```python
from build123d import *

# Parameters (mm, degrees)
F1_W     = 450
F1_H     = 450
F2_DEPTH = 25
F3_W     = 50
F3_H     = 50
F4_DEPTH = 450
F6_DEPTH = 25
F8_DEPTH = 25


with BuildPart() as f2:
    # F1 (on offset) → F2 (new body)
    with BuildSketch(Plane.XY.offset(450)):
        Rectangle(F1_W, F1_H)
    extrude(amount=F2_DEPTH)

    # F3 (on face) → F4 (join, through all)
    with BuildSketch(Plane(origin=(0, 0, 450), x_dir=(1, 0, 0), z_dir=(0, 0, -1))):
        with Locations((-200, -200)):
            Rectangle(F3_W, F3_H)
        with Locations((-200, 200)):
            Rectangle(F3_W, F3_H)
        with Locations((200, -200)):
            Rectangle(F3_W, F3_H)
        with Locations((200, 200)):
            Rectangle(F3_W, F3_H)
    extrude(amount=F4_DEPTH)

    # F5 (on face) → F6 (join)
    with BuildSketch(Plane.XZ.offset(225)):
        with BuildLine():
            Line((-277.210476888, 871.5779445495), (-225, 475))
            Line((-225, 475), (-174.568551971, 475))
            Line((-174.568551971, 475), (-219.5097934393, 816.3626197141))
            ThreePointArc((-219.5097934393, 816.3626197141), (0, 864.4554478408), (219.5097934393, 816.3626197141))
            Line((219.5097934393, 816.3626197141), (174.568551971, 475))
            Line((174.568551971, 475), (225, 475))
            Line((225, 475), (277.210476888, 871.5779445495))
            ThreePointArc((277.210476888, 871.5779445495), (0, 939.4554478408), (-277.210476888, 871.5779445495))
        make_face()
    extrude(amount=-F6_DEPTH)

    # F7 (on face) → F8 (join)
    with BuildSketch(Plane.XZ.offset(225)):
        with BuildLine():
            ThreePointArc((12.5, 864.3066172212), (0, 864.4554478408), (-12.5, 864.3066172212))
            Line((-12.5, 864.3066172212), (-12.5, 475))
            Line((-12.5, 475), (12.5, 475))
            Line((12.5, 475), (12.5, 864.3066172212))
        make_face()
        with BuildLine():
            Line((-140.2890822889, 871.5293721566), (-112.561047452, 475))
            Line((-112.561047452, 475), (-87.5, 475))
            Line((-87.5, 475), (-115.6574592783, 877.6704277765))
            ThreePointArc((-115.6574592783, 877.6704277765), (-127.9664582867, 874.5725752089), (-140.2890822889, 871.5293721566))
        make_face()
        with BuildLine():
            Line((87.5, 475), (112.561047452, 475))
            Line((112.561047452, 475), (140.2890822889, 871.5293721566))
            ThreePointArc((140.2890822889, 871.5293721566), (127.9664582867, 874.5725752089), (115.6574592783, 877.6704277765))
            Line((115.6574592783, 877.6704277765), (87.5, 475))
        make_face()
    extrude(amount=-F8_DEPTH)


solid = f2.part
```
Part model, mm, in its own coordinate system. A direction names the side the tool comes from. Round coordinates to 2 decimals unless told otherwise and drop trailing zeros. Loops run counter-clockwise (first coordinate to the right, second up) from the corner with the lowest first, then second, coordinate; pieces in that order, holes last. Notation, with made-up numbers: (3.5, 2.25) -> (21.5, 2.25) arc R33 ccw to (21.5, 33.25) -> close; hole circle Ø11 at (71, 3.25). An arc over 180 degrees is marked (long way). Use one line per item in the form item = value. Start each with the question number.
Item 1: Band-saw the part on D-D (y = 127.5). List the corners of the cut face in (x, z).
Item 2: Drop flat-ended pins along their axis: pin 1 Ø12 at (x, y) = (186, -64.5) entering from -Z; pin 2 Ø25 at (y, z) = (-201, 234) entering from -X; pin 3 Ø8 at (x, y) = (205, 165) entering from +Z. Give the stop position or say it passes through.
Item 3: Tool access for faces 4 (the flat face through (-100.495, -212.675, 660.841)), 5 (the flat face through (200, -175, 228)), 6 (the flat face through (-4, -200, 762)): list every direction of +Z, -Z, +X, -X, +Y, -Y with a clear straight run to the whole face (end or side of a thin tool).
Item 4: Two-plate mould, pull along X, no slides. Class faces 1 (the flat face through (225, -184, 272)), 2 (the flat face through (-200, -175, 228)), 3 (the flat face through (-175, 200, 228)): released by +X, released by -X, zero draft, split by the parting line, or undercut.
Item 5: Band-saw the part on B-B (x = -103). List the corners of the cut face in (y, z).
Item 6: Drill centre lines: line 1 along Y through (x, z) = (185, 124); line 2 along Z through (x, y) = (-72, -131). Where is each one in solid material? Low to high.
Item 7: Band-saw the part on C-C (z = 673.5). List the corners of the cut face in (x, y).
Item 8: Band-saw the part on A-A (z = 63). List the corners of the cut face in (x, y).
Data:
q1.outline = (-225, 450) -> (225, 450) -> (225, 475) -> (-225, 475) -> close
q2.pin_1 = 450
q2.pin_2 = -225
q2.pin_3 = 475
q3.face_4 = +Y, -Y
q3.face_5 = -Z, +X, -X
q3.face_6 = +Z, +X, -X, +Y
q4.face_1 = released by +X
q4.face_2 = zero draft
q4.face_3 = undercut
q5.outline = (-225, 450) -> (225, 450) -> (225, 475) -> (-200, 475) -> (-200, 696.66) -> (-225, 696.66) -> close; (-225, 854.25) -> (-200, 854.25) -> (-200, 930.55) -> (-225, 930.55) -> close
q6.line_1 = -225 to -175, 175 to 225
q6.line_2 = 450 to 475
q7.outline = (-251.13, -225) -> (-200.7, -225) -> (-200.7, -200) -> (-251.13, -200) -> close; (-126.44, -225) -> (-101.38, -225) -> (-101.38, -200) -> (-126.44, -200) -> close; (-12.5, -225) -> (12.5, -225) -> (12.5, -200) -> (-12.5, -200) -> close; (101.38, -225) -> (126.44, -225) -> (126.44, -200) -> (101.38, -200) -> close; (200.7, -225) -> (251.13, -225) -> (251.13, -200) -> (200.7, -200) -> close
q8.outline = (-225, -225) -> (-175, -225) -> (-175, -175) -> (-225, -175) -> close; (-225, 175) -> (-175, 175) -> (-175, 225) -> (-225, 225) -> close; (175, -225) -> (225, -225) -> (225, -175) -> (175, -175) -> close; (175, 175) -> (225, 175) -> (225, 225) -> (175, 225) -> close
